Design review of the part shown in the three views and the two pictorial views. Dimensions are in mm from the part's minimum x, y and z. A direction names the side the tool comes from. Give positions to 0.01 mm unless a question says otherwise; leave off trailing zeros. Loops run counter-clockwise (first coordinate to the right, second up) from the corner with the lowest first, then second, coordinate; pieces in that order, holes last. Notation, with made-up numbers: M 62,28 L 76,28 A17 ccw 76,55 Z; hole C 56,-29.75 d1. An arc over 180 degrees is marked long. Return JSON: item names as keys, results as strings. Group by question number.
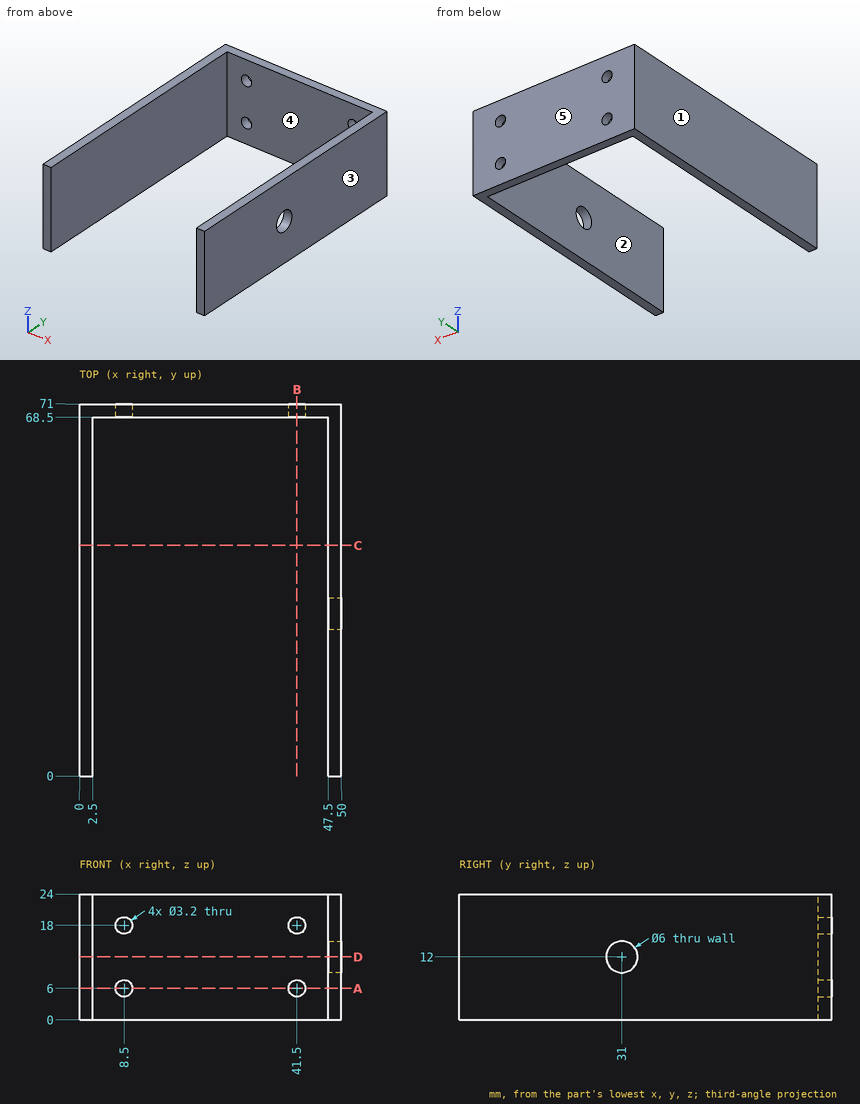
(1) Mouldability with a two-part tool opening along X and no side actions: class the marked faces 3, 4 and 5 as released by +X, released by -X, zero draft, split by the parting line, or undercut.
(2) Add section A-A (z = 6). Write out the cut boundary in (x, y), and give its area (4 significant figures).
(3) For probe 1 along X at (y, z) = (70.45, 18); probe 2 along Z at (x, y) = (41.5, 70.05); probe 3 along X at (y, z) = (45.5, 13.25), list the stretches that pass through material, from the lowest coordinate up.
(4) Add section D-D (z = 12). Write out the cut boundary in (x, y).
(5) For pin 1 (8 mm diameter, centred on x = 29.5, z = 15, fed in from -Y); pin 2 (3 mm diameter, centred on x = 41.5, z = 18, fed in from +Y), all flat-tipped, find the tip position at first contact; note any pin that passes through.
(6) Add section C-C (y = 44). Write out the cut boundary in (x, z).
(7) For the marked faces 1 and 2, list the 3-axis set-ups (+Z, -Z, +X, -X, +Y, -Y) from which the entire face can be reached by the end or side of a thin tool; tool diameter is ignored.
(8) Add section B-B (x = 41.5). Write out the cut boundary in (y, z), and give its area (3 significant figures).
Verdict:
{
 "1": {"face 3": "released by +X", "face 4": "undercut", "face 5": "zero draft"},
 "2": {"outline": "M 0,0 L 2.5,0 L 2.5,68.5 L 6.9,68.5 L 6.9,71 L 0,71 Z; M 10.1,68.5 L 39.9,68.5 L 39.9,71 L 10.1,71 Z; M 43.1,68.5 L 47.5,68.5 L 47.5,0 L 50,0 L 50,71 L 43.1,71 Z", "area": "451.5 mm²"},
 "3": {"probe 1": "x = 0 to 6.9, 10.1 to 39.9, 43.1 to 50", "probe 2": "z = 0 to 4.4, 7.6 to 16.4, 19.6 to 24", "probe 3": "x = 0 to 2.5, 47.5 to 50"},
 "4": {"outline": "M 0,0 L 2.5,0 L 2.5,68.5 L 47.5,68.5 L 47.5,34 L 50,34 L 50,71 L 0,71 Z; M 47.5,0 L 50,0 L 50,28 L 47.5,28 Z"},
 "5": {"pin 1": "stops at y = 68.5", "pin 2": "passes through"},
 "6": {"outline": "M 0,0 L 2.5,0 L 2.5,24 L 0,24 Z; M 47.5,0 L 50,0 L 50,24 L 47.5,24 Z"},
 "7": {"face 1": "+Z, -Z, -X, +Y, -Y", "face 2": "+Z, -Z, -Y"},
 "8": {"outline": "M 68.5,0 L 71,0 L 71,4.4 L 68.5,4.4 Z; M 68.5,7.6 L 71,7.6 L 71,16.4 L 68.5,16.4 Z; M 68.5,19.6 L 71,19.6 L 71,24 L 68.5,24 Z", "area": "44.0 mm²"}
}
